Here's how the part is built. I have some questions about the finished solid (model axes, mm). A direction names the side the tool comes from. Give positions to 0.01 mm unless a question says otherwise; leave off trailing zeros. Loops run counter-clockwise (first coordinate to the right, second up) from the corner with the lowest first, then second, coordinate; pieces in that order, holes last. Notation, with made-up numbers: (59, 3.5) - (97, 3.5) arc R19 ccw to (97, 13.5) - close; hole circle Ø11 at (46.25, 36). An arc over 180 degrees is marked (long way). Use a Markdown table: item, result.
from build123d import *

# Parameters (mm, degrees)
SKETCH2_W           = 15
SKETCH2_H           = 15
BOSS_EXTRUDE1_DEPTH = 2
SKETCH3_R           = 3.5
SKETCH3_R_2         = 2.5
BOSS_EXTRUDE2_DEPTH = 10
FILLET1_R           = 1
FILLET2_R           = 1


with BuildPart() as part:
    # Sketch2 → Boss-Extrude1 (new body)
    with BuildSketch(Plane(origin=(0, 0, 0), x_dir=(1, 0, 0), z_dir=(0, 1, 0))):
        Rectangle(SKETCH2_W, SKETCH2_H)
    extrude(amount=BOSS_EXTRUDE1_DEPTH)

    # Sketch3 → Boss-Extrude2 (add)
    with BuildSketch(Plane.XZ):
        with Locations(Location((0, 0, 0), (0, 0, 270))):
            Circle(SKETCH3_R)
        with Locations(Location((0, 0, 0), (0, 0, 270))):
            Circle(SKETCH3_R_2, mode=Mode.SUBTRACT)
    extrude(amount=BOSS_EXTRUDE2_DEPTH)

    # Fillet1
    fillet1_edges = [part.edges().sort_by_distance(p)[0] for p in [
        (0, 0, 3.5),
    ]]
    fillet(fillet1_edges, radius=FILLET1_R)

    # Fillet2
    fillet2_edges = [part.edges().sort_by_distance(p)[0] for p in [
        (0, 0, 2.5),
    ]]
    fillet(fillet2_edges, radius=FILLET2_R)


solid = part.part
(1) On a 3-axis mill with a long thin cutter (end or side, diameter ignored), from which of +Z, -Z, +X, -X, +Y, -Y can I reach the whole of each face in a straight line? I mean faces 1 (the face through (-3.4, 0, -3.4)), 2 (the face through (0, 2, 0)). Say none if no direction works.
A:
| item | result |
|---|---|
| face 1 | -Y |
| face 2 | +Z, -Z, +X, -X, +Y |
(2) Suppose I cut it at C-C on y = -0.5. Write out the boundary of the cut face in (x, z).
A:
| item | result |
|---|---|
| outline | circle Ø7.27 at (0, 0); hole circle Ø4.73 at (0, 0) |
(3) Suppose I cut it at A-A on z = 0. Write out the boundary of the cut face in (x, y), plus the area to 3 significant figures.
A:
| item | result |
|---|---|
| outline | (-7.5, 0) - (-4.5, 0) arc R1 cw to (-3.5, -1) - (-3.5, -10) - (-2.5, -10) - (-2.5, -1) arc R1 cw to (-1.5, 0) - (1.5, 0) arc R1 cw to (2.5, -1) - (2.5, -10) - (3.5, -10) - (3.5, -1) arc R1 cw to (4.5, 0) - (7.5, 0) - (7.5, 2) - (-7.5, 2) - close |
| area | 50.9 mm2 |
(4) We'd pull the mould along X, two halves only. Please class faces 3 (the face through (-3.417, -5.437, 0.759)), 4 (the face through (-2, -10, -2)), 5 (the face through (-2.44, -5.44, 0.54)), 6 (the face through (0, 0, 0)): pulls with the +X half, pulls with the -X half, needs draft (parallel to the pull), parting line crosses it, or undercut.
A:
| item | result |
|---|---|
| face 3 | parting line crosses it |
| face 4 | needs draft |
| face 5 | undercut |
| face 6 | undercut |
(5) Will these pins go through, and if not, where does the flat tip stop? pin 1 (2 mm diameter, centred on y = -3, z = -2, fed in from +X); pin 2 (3 mm diameter, centred on x = 0, z = 0, fed in from -Y); pin 3 (2 mm diameter, centred on x = 2, y = -7.5, fed in from +Z).
A:
| item | result |
|---|---|
| pin 1 | x = 3.35 |
| pin 2 | y = 0 |
| pin 3 | z = 3.35 |
(6) If I drill on line 1 (X direction, y = -5, z = 0); line 2 (Y direction, x = -4, z = 2.75); line 3 (X direction, y = -7, z = -2), over which ranges is the centre line in solid material (lowest first)?
A:
| item | result |
|---|---|
| line 1 | -3.5 to -2.5, 2.5 to 3.5 |
| line 2 | 0 to 2 |
| line 3 | -2.87 to -1.5, 1.5 to 2.87 |
(7) Suppose I cut it at D-D on x = -4.75. Write out the boundary of the cut face in (y, z), plus the area to 3 significant figures.
A:
| item | result |
|---|---|
| outline | (0, -7.5) - (2, -7.5) - (2, 7.5) - (0, 7.5) - close |
| area | 30.0 mm2 |
(8) Suppose I cut it at B-B on x = 0. Write out the boundary of the cut face in (y, z), plus the area to 3 significant figures.
A:
| item | result |
|---|---|
| outline | (-10, -3.5) - (-1, -3.5) arc R1 cw to (0, -4.5) - (0, -7.5) - (2, -7.5) - (2, 7.5) - (0, 7.5) - (0, 4.5) arc R1 cw to (-1, 3.5) - (-10, 3.5) - (-10, 2.5) - (-1, 2.5) arc R1 cw to (0, 1.5) - (0, -1.5) arc R1 cw to (-1, -2.5) - (-10, -2.5) - close |
| area | 50.9 mm2 |
